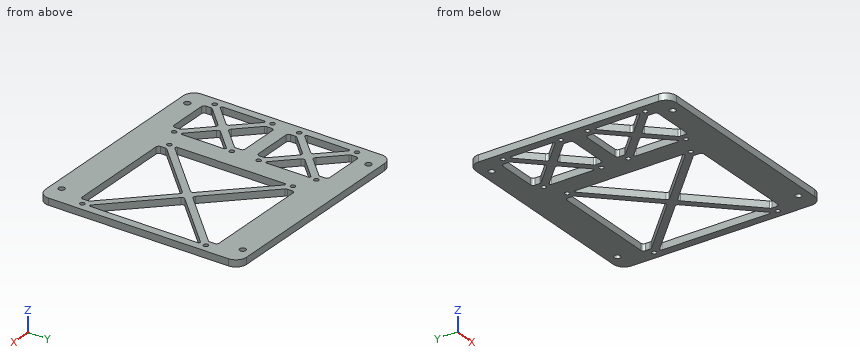
from build123d import *

# Parameters (mm, degrees)
SKETCH_1_W          = 150
SKETCH_1_H          = 162
EXTRUDE_1_DEPTH     = 5
HOLE_WIZARD_M3_1_D  = 3.4
HOLE_WIZARD_M4_1_D  = 4.5
CUT_EXTRUDE_2_DEPTH = 221.837043994
FILLET_8_R          = 8
FILLET_11_R         = 2
FILLET_13_R         = 1


with BuildPart() as part:
    # ｽｹｯﾁ1 → ﾎﾞｽ - 押し出し1 (new body)
    with BuildSketch(Plane(origin=(0, 0, 0), x_dir=(0, 1, 0), z_dir=(0, 0, 1))):
        with Locations((75, 81)):
            Rectangle(SKETCH_1_W, SKETCH_1_H)
    extrude(amount=EXTRUDE_1_DEPTH)

    # M3 すきま穴1 (through all)
    with Locations(Plane.XY.offset(5)):
        with Locations((-156, 65), (-6, 121.04), (-6, 28.96), (-98.08, 28.96), (-113, 128), (-98.08, 121.04), (-156, 85), (-113, 85), (-156, 128), (-113, 65), (-156, 22), (-113, 22)):
            Hole(HOLE_WIZARD_M3_1_D / 2)

    # M4 すきま穴1 (through all)
    with Locations(Plane.XY.offset(5)):
        with Locations((-147.5, 142.5), (-14.5, 142.5), (-14.5, 7.5), (-147.5, 7.5)):
            Hole(HOLE_WIZARD_M4_1_D / 2)

    # ｽｹｯﾁ6 → ｶｯﾄ - 押し出し2 (cut, through all)
    with BuildSketch(Plane.XY.offset(5)):
        Polygon((-93.08, 23.96), (-93.08, 30.424466094), (-52.04, 71.464466094), (-11, 30.424466094), (-11, 23.96), align=None)
        Polygon((-98.08, 116.04), (-96.615533906, 116.04), (-55.575533906, 75), (-96.615533906, 33.96), (-98.08, 33.96), align=None)
        Polygon((-93.08, 126.04), (-11, 126.04), (-11, 119.575533906), (-52.04, 78.535533906), (-93.08, 119.575533906), align=None)
        Polygon((-151, 133), (-118, 133), (-118, 126.535533906), (-134.5, 110.035533906), (-151, 126.535533906), align=None)
        Polygon((-151, 70), (-118, 70), (-118, 63.535533906), (-134.5, 47.035533906), (-151, 63.535533906), align=None)
        Polygon((-151, 17), (-118, 17), (-118, 23.464466094), (-134.5, 39.964466094), (-151, 23.464466094), align=None)
        Polygon((-154.535533906, 123), (-138.035533906, 106.5), (-154.535533906, 90), (-156, 90), (-156, 123), align=None)
        Polygon((-151, 86.464466094), (-134.5, 102.964466094), (-118, 86.464466094), (-118, 80), (-151, 80), align=None)
        Polygon((-154.535533906, 60), (-138.035533906, 43.5), (-154.535533906, 27), (-156, 27), (-156, 60), align=None)
        Polygon((-114.464466094, 123), (-113, 123), (-113, 90), (-114.464466094, 90), (-130.964466094, 106.5), align=None)
        Polygon((-130.964466094, 43.5), (-114.464466094, 60), (-113, 60), (-113, 27), (-114.464466094, 27), align=None)
        Polygon((-7.464466094, 33.96), (-6, 33.96), (-6, 116.04), (-7.464466094, 116.04), (-48.504466094, 75), align=None)
    extrude(amount=-CUT_EXTRUDE_2_DEPTH, mode=Mode.SUBTRACT)

    # ﾌｨﾚｯﾄ8
    fillet_8_edges = [part.edges().sort_by_distance(p)[0] for p in [
        (-162, 0, 2.5),
        (-162, 150, 2.5),
        (0, 150, 2.5),
        (0, 0, 2.5),
    ]]
    fillet(fillet_8_edges, radius=FILLET_8_R)

    # ﾌｨﾚｯﾄ11
    fillet_11_edges = [part.edges().sort_by_distance(p)[0] for p in [
        (-130.964466094, 43.5, 2.5),
        (-151, 17, 2.5),
        (-151, 23.464466094, 2.5),
        (-134.5, 39.964466094, 2.5),
        (-118, 23.464466094, 2.5),
        (-118, 17, 2.5),
        (-138.035533906, 43.5, 2.5),
        (-55.575533906, 75, 2.5),
        (-151, 80, 2.5),
        (-151, 86.464466094, 2.5),
        (-134.5, 102.964466094, 2.5),
        (-118, 86.464466094, 2.5),
        (-118, 80, 2.5),
        (-138.035533906, 106.5, 2.5),
        (-118, 133, 2.5),
        (-118, 126.535533906, 2.5),
        (-134.5, 110.035533906, 2.5),
        (-151, 126.535533906, 2.5),
        (-151, 133, 2.5),
        (-118, 70, 2.5),
        (-118, 63.535533906, 2.5),
        (-134.5, 47.035533906, 2.5),
        (-151, 63.535533906, 2.5),
        (-151, 70, 2.5),
        (-93.08, 119.575533906, 2.5),
        (-93.08, 126.04, 2.5),
        (-11, 126.04, 2.5),
        (-11, 119.575533906, 2.5),
        (-52.04, 78.535533906, 2.5),
        (-93.08, 30.424466094, 2.5),
        (-52.04, 71.464466094, 2.5),
        (-11, 30.424466094, 2.5),
        (-11, 23.96, 2.5),
        (-93.08, 23.96, 2.5),
        (-48.504466094, 75, 2.5),
        (-130.964466094, 106.5, 2.5),
    ]]
    fillet(fillet_11_edges, radius=FILLET_11_R)

    # ﾌｨﾚｯﾄ13
    fillet_13_edges = [part.edges().sort_by_distance(p)[0] for p in [
        (-113, 27, 2.5),
        (-114.464466094, 27, 2.5),
        (-114.464466094, 60, 2.5),
        (-113, 60, 2.5),
        (-156, 60, 2.5),
        (-154.535533906, 60, 2.5),
        (-154.535533906, 27, 2.5),
        (-156, 27, 2.5),
        (-96.615533906, 33.96, 2.5),
        (-98.08, 33.96, 2.5),
        (-98.08, 116.04, 2.5),
        (-96.615533906, 116.04, 2.5),
        (-156, 90, 2.5),
        (-156, 123, 2.5),
        (-154.535533906, 123, 2.5),
        (-154.535533906, 90, 2.5),
        (-6, 116.04, 2.5),
        (-6, 33.96, 2.5),
        (-7.464466094, 33.96, 2.5),
        (-7.464466094, 116.04, 2.5),
        (-114.464466094, 90, 2.5),
        (-114.464466094, 123, 2.5),
        (-113, 123, 2.5),
        (-113, 90, 2.5),
    ]]
    fillet(fillet_13_edges, radius=FILLET_13_R)


solid = part.part
The model under review builds one solid part; all positions refer to its coordinate system, in mm. Coordinates: 2 decimals unless noted, no trailing zeros. Loops run counter-clockwise (first coordinate to the right, second up) from the corner with the lowest first, then second, coordinate; pieces in that order, holes last. Notation, with made-up numbers: M -27,73 L 14,73 A11 cw 14,81 Z; hole C 41.5,88.5 d7. An arc over 180 degrees is marked long. Put each result on its own line as item: value. Start each with the question number.
Q1. Wall thickness on line 1 (X direction, y = 142.5, z = 1.9); line 2 (Y direction, x = -111.5, z = 0.2); line 3 (Y direction, x = -63, z = 2.7): over which ranges is each line inside the solid? List them lowest first.
Q2. Add section A-A (x = -30). Write out the cut boundary in (y, z), and give its area (3 significant figures).
Q3. Add section C-C (x = -123.5). Write out the cut boundary in (y, z).
Q4. Add section B-B (z = 1.55). Count the separate pieces of the cut face and the enclosed holes in it, and give its area (3 significant figures).
Answers:
1. line 1: x = -161.98 to -149.75, -145.25 to -16.75, -12.25 to -0.02
1. line 2: y = 0 to 21.2, 22.8 to 64.2, 65.8 to 84.2, 85.8 to 127.2, 128.8 to 150
1. line 3: y = 0 to 23.96, 60.5 to 67.58, 82.42 to 89.5, 126.04 to 150
2. outline: M 0,0 L 23.96,0 L 23.96,5 L 0,5 Z; M 49.42,0 L 56.5,0 L 56.5,5 L 49.42,5 Z; M 93.5,0 L 100.58,0 L 100.58,5 L 93.5,5 Z; M 126.04,0 L 150,0 L 150,5 L 126.04,5 Z
2. area: 310 mm^2
3. outline: M 0,0 L 17,0 L 17,5 L 0,5 Z; M 28.96,0 L 36.04,0 L 36.04,5 L 28.96,5 Z; M 50.96,0 L 58.04,0 L 58.04,5 L 50.96,5 Z; M 70,0 L 80,0 L 80,5 L 70,5 Z; M 91.96,0 L 99.04,0 L 99.04,5 L 91.96,5 Z; M 113.96,0 L 121.04,0 L 121.04,5 L 113.96,5 Z; M 133,0 L 150,0 L 150,5 L 133,5 Z
4. separate pieces: 1
4. enclosed holes: 28
4. area: 12,800 mm^2
